Geometry: final body of the model. Coordinates: model frame, mm. A direction names the side the tool comes from. Give positions to 0.01 mm unless a question says otherwise; leave off trailing zeros. Loops run counter-clockwise (first coordinate to the right, second up) from the corner with the lowest first, then second, coordinate; pieces in that order, holes last. Notation, with made-up numbers: (-34, 59) -> (14, 59) arc R11 ccw to (14, 69) -> close; hole circle Ø7 at (-38, -27). An arc over 180 degrees is marked (long way). Answer in a Markdown table with one row per item. Add a question column.
from build123d import *

# Parameters (mm, degrees)
CYLINDER873_R               = 3.1
CYLINDER873_DEPTH           = 5
CYLINDER873_ROLL_ANGLE      = 90
CYLINDER872_R               = 5.6
CYLINDER872_DEPTH           = 4.5
CYLINDER872_ROLL_ANGLE      = 90
CYLINDER871_R               = 5.6
CYLINDER871_DEPTH           = 4
CYLINDER871_ROLL_ANGLE      = 90
CYLINDER870_R               = 3.5
CYLINDER870_DEPTH           = 14
CYLINDER870_ROLL_ANGLE      = 90
CYLINDER866_R               = 1.6
CYLINDER866_DEPTH           = 20
CYLINDER866_ROLL_ANGLE      = 90
CYLINDER869_R               = 2.1
CYLINDER869_DEPTH           = 20
CYLINDER869_ROLL_ANGLE      = 90
CYLINDER868_R               = 1.6
CYLINDER868_DEPTH           = 6.75
CYLINDER868_ROLL_ANGLE      = 90
CYLINDER867_R               = 2.8
CYLINDER867_DEPTH           = 10
CYLINDER867_ROLL_ANGLE      = 90
BOX542_W                    = 16
BOX542_H                    = 13
BOX542_DEPTH                = 14
BOX539_W                    = 12
BOX539_H                    = 7.5
BOX539_DEPTH                = 8
BOX538_W                    = 12
BOX538_H                    = 13.75
BOX538_DEPTH                = 12
BOX540_W                    = 30
BOX540_H                    = 3.75
BOX540_DEPTH                = 10
BOX541_W                    = 22
BOX541_H                    = 3.75
BOX541_DEPTH                = 14
FILLET352_R                 = 4
FILLET353_R                 = 3
FILLET354_R                 = 3
FILLET355_R                 = 4
FILLET356_R                 = 3
BOX543_W                    = 16
BOX543_H                    = 3.75
BOX543_DEPTH                = 2
CHAMFER102_SIZE             = 1.99
CYLINDER877_R               = 2.8
CYLINDER877_DEPTH           = 11
CYLINDER877_ROLL_ANGLE      = 89.99995
CYLINDER877_PITCH_ANGLE     = -5e-06
CYLINDER877_PLACEMENT_ANGLE = -10.999997
BOX545_W                    = 1.9
BOX545_H                    = 10
BOX545_DEPTH                = 8


with BuildPart() as cylinder1034:
    # Cylinder873 → Cylinder873 (new body)
    with BuildSketch(Plane.XY):
        Circle(CYLINDER873_R)
    extrude(amount=CYLINDER873_DEPTH)


with BuildPart() as cylinder1034_1:
    # Cylinder873 roll: moved
    add(cylinder1034.part.rotate(Axis((0, 0, 0), (1, 0, 0)), CYLINDER873_ROLL_ANGLE))


with BuildPart() as cylinder1034_2:
    # Cylinder873 placement: moved
    add(cylinder1034_1.part.moved(Location((49.5, 49.75, -13))))


with BuildPart() as cylinder1033:
    # Cylinder872 → Cylinder872 (new body)
    with BuildSketch(Plane.XY):
        Circle(CYLINDER872_R)
    extrude(amount=CYLINDER872_DEPTH)


with BuildPart() as cylinder1033_1:
    # Cylinder872 roll: moved
    add(cylinder1033.part.rotate(Axis((0, 0, 0), (1, 0, 0)), CYLINDER872_ROLL_ANGLE))


with BuildPart() as cylinder1033_2:
    # Cylinder872 placement: moved
    add(cylinder1033_1.part.moved(Location((38, 53.5, -11))))


with BuildPart() as cylinder1032:
    # Cylinder871 → Cylinder871 (new body)
    with BuildSketch(Plane.XY):
        Circle(CYLINDER871_R)
    extrude(amount=CYLINDER871_DEPTH)


with BuildPart() as cylinder1032_1:
    # Cylinder871 roll: moved
    add(cylinder1032.part.rotate(Axis((0, 0, 0), (1, 0, 0)), CYLINDER871_ROLL_ANGLE))


with BuildPart() as cylinder1032_2:
    # Cylinder871 placement: moved
    add(cylinder1032_1.part.moved(Location((38, 43.75, -11))))


with BuildPart() as fusion560:
    # Cylinder870 → Cylinder870 (new body)
    with BuildSketch(Plane.XY):
        Circle(CYLINDER870_R)
    extrude(amount=CYLINDER870_DEPTH)


with BuildPart() as fusion560_1:
    # Cylinder870 roll: moved
    add(fusion560.part.rotate(Axis((0, 0, 0), (1, 0, 0)), CYLINDER870_ROLL_ANGLE))


with BuildPart() as fusion560_2:
    # Cylinder870 placement: moved
    add(fusion560_1.part.moved(Location((38, 53.5, -11))))

    # Fusion560: union Cylinder1033, Cylinder1032
    add(cylinder1033_2.part)
    add(cylinder1032_2.part)


with BuildPart() as fusion560_3:
    # Fusion560 placement: moved
    add(fusion560_2.part.moved(Location((-1, 0, 0))))


with BuildPart() as cylinder1027:
    # Cylinder866 → Cylinder866 (new body)
    with BuildSketch(Plane.XY):
        Circle(CYLINDER866_R)
    extrude(amount=CYLINDER866_DEPTH)


with BuildPart() as cylinder1027_1:
    # Cylinder866 roll: moved
    add(cylinder1027.part.rotate(Axis((0, 0, 0), (1, 0, 0)), CYLINDER866_ROLL_ANGLE))


with BuildPart() as cylinder1027_2:
    # Cylinder866 placement: moved
    add(cylinder1027_1.part.moved(Location((49.5, 56.5, -13))))


with BuildPart() as cylinder1030:
    # Cylinder869 → Cylinder869 (new body)
    with BuildSketch(Plane.XY):
        Circle(CYLINDER869_R)
    extrude(amount=CYLINDER869_DEPTH)


with BuildPart() as cylinder1030_1:
    # Cylinder869 roll: moved
    add(cylinder1030.part.rotate(Axis((0, 0, 0), (1, 0, 0)), CYLINDER869_ROLL_ANGLE))


with BuildPart() as cylinder1030_2:
    # Cylinder869 placement: moved
    add(cylinder1030_1.part.moved(Location((45.5, 56.5, -26))))


with BuildPart() as fusion559:
    # Cylinder868 → Cylinder868 (new body)
    with BuildSketch(Plane.XY):
        Circle(CYLINDER868_R)
    extrude(amount=CYLINDER868_DEPTH)


with BuildPart() as fusion559_1:
    # Cylinder868 roll: moved
    add(fusion559.part.rotate(Axis((0, 0, 0), (1, 0, 0)), CYLINDER868_ROLL_ANGLE))


with BuildPart() as fusion559_2:
    # Cylinder868 placement: moved
    add(fusion559_1.part.moved(Location((28.5, 56.5, -11))))

    # Fusion559: union Cylinder1027, Cylinder1030
    add(cylinder1027_2.part)
    add(cylinder1030_2.part)


with BuildPart() as cylinder1028:
    # Cylinder867 → Cylinder867 (new body)
    with BuildSketch(Plane.XY):
        Circle(CYLINDER867_R)
    extrude(amount=CYLINDER867_DEPTH)


with BuildPart() as cylinder1028_1:
    # Cylinder867 roll: moved
    add(cylinder1028.part.rotate(Axis((0, 0, 0), (1, 0, 0)), CYLINDER867_ROLL_ANGLE))


with BuildPart() as cylinder1028_2:
    # Cylinder867 placement: moved
    add(cylinder1028_1.part.moved(Location((28.5, 49.75, -11))))


with BuildPart() as cube733:
    # Box542 → Box542 (new body)
    with BuildSketch(Plane(origin=(29.5, 39.75, -18), x_dir=(1, 0, 0), z_dir=(0, 0, 1))):
        with Locations((8, 6.5)):
            Rectangle(BOX542_W, BOX542_H)
    extrude(amount=BOX542_DEPTH)


with BuildPart() as cube730:
    # Box539 → Box539 (new body)
    with BuildSketch(Plane(origin=(389.5, 41.75, -32), x_dir=(1, 0, 0), z_dir=(0, 0, 1))):
        with Locations((6, 3.75)):
            Rectangle(BOX539_W, BOX539_H)
    extrude(amount=BOX539_DEPTH)


with BuildPart() as cut892:
    # Box538 → Box538 (new body)
    with BuildSketch(Plane(origin=(389.5, 39.75, -32), x_dir=(1, 0, 0), z_dir=(0, 0, 1))):
        with Locations((6, 6.875)):
            Rectangle(BOX538_W, BOX538_H)
    extrude(amount=BOX538_DEPTH)

    # Cut663: cut Cube730
    add(cube730.part, mode=Mode.SUBTRACT)


with BuildPart() as fusion556:
    # Box540 → Box540 (new body)
    with BuildSketch(Plane(origin=(373.5, 49.75, -20), x_dir=(1, 0, 0), z_dir=(0, 0, 1))):
        with Locations((15, 1.875)):
            Rectangle(BOX540_W, BOX540_H)
    extrude(amount=BOX540_DEPTH)

    # Fusion556: union Cut892
    add(cut892.part)


with BuildPart() as fusion556_1:
    # Fusion556 placement: moved
    add(fusion556.part.moved(Location((-350, 0, 2))))


with BuildPart() as fillet356:
    # Box541 → Box541 (new body)
    with BuildSketch(Plane(origin=(23.5, 49.75, -18), x_dir=(1, 0, 0), z_dir=(0, 0, 1))):
        with Locations((11, 1.875)):
            Rectangle(BOX541_W, BOX541_H)
    extrude(amount=BOX541_DEPTH)

    # Fusion557: union Fusion556
    add(fusion556_1.part)

    # Fusion558: union Cube733
    add(cube733.part)

    # Cut664: cut Cylinder1028
    add(cylinder1028_2.part, mode=Mode.SUBTRACT)

    # Cut665: cut Fusion559
    add(fusion559_2.part, mode=Mode.SUBTRACT)

    # Cut666: cut Fusion560
    add(fusion560_3.part, mode=Mode.SUBTRACT)

    # Fillet352
    fillet352_edges = [fillet356.edges().sort_by_distance(p)[0] for p in [
        (51.5, 40.75, -30),
        (51.5, 51.375, -30),
        (39.5, 40.75, -30),
        (39.5, 51.375, -30),
    ]]
    fillet(fillet352_edges, radius=FILLET352_R)

    # Fillet353
    fillet353_edges = [fillet356.edges().sort_by_distance(p)[0] for p in [
        (49.5, 49.75, -8),
        (48.5, 39.75, -18),
    ]]
    fillet(fillet353_edges, radius=FILLET353_R)

    # Fillet354
    fillet354_edges = [fillet356.edges().sort_by_distance(p)[0] for p in [
        (48.5, 49.75, -18),
    ]]
    fillet(fillet354_edges, radius=FILLET354_R)

    # Cut667: cut Cylinder1034
    add(cylinder1034_2.part, mode=Mode.SUBTRACT)

    # Fillet355
    fillet355_edges = [fillet356.edges().sort_by_distance(p)[0] for p in [
        (23.5, 51.625, -18),
        (23.5, 51.625, -4),
    ]]
    fillet(fillet355_edges, radius=FILLET355_R)

    # Fillet356
    fillet356_edges = [fillet356.edges().sort_by_distance(p)[0] for p in [
        (29.5, 44.75, -18),
        (45.5, 46.625, -4),
        (29.5, 44.75, -4),
    ]]
    fillet(fillet356_edges, radius=FILLET356_R)


with BuildPart() as chamfer102:
    # Box543 → Box543 (new body)
    with BuildSketch(Plane(origin=(37.5, 49.75, -20), x_dir=(1, 0, 0), z_dir=(0, 0, 1))):
        with Locations((8, 1.875)):
            Rectangle(BOX543_W, BOX543_H)
    extrude(amount=BOX543_DEPTH)

    # Chamfer102
    chamfer102_edges = [chamfer102.edges().sort_by_distance(p)[0] for p in [
        (37.5, 51.625, -20),
        (53.5, 51.625, -20),
    ]]
    chamfer(chamfer102_edges, length=CHAMFER102_SIZE)


with BuildPart() as cylinder1038:
    # Cylinder877 → Cylinder877 (new body)
    with BuildSketch(Plane.XY):
        Circle(CYLINDER877_R)
    extrude(amount=CYLINDER877_DEPTH)


with BuildPart() as cylinder1038_1:
    # Cylinder877 roll: moved
    add(cylinder1038.part.rotate(Axis((0, 0, 0), (1, 0, 0)), CYLINDER877_ROLL_ANGLE))


with BuildPart() as cylinder1038_2:
    # Cylinder877 pitch: moved
    add(cylinder1038_1.part.rotate(Axis((0, 0, 0), (0, 1, 0)), CYLINDER877_PITCH_ANGLE))


with BuildPart() as cylinder1038_3:
    # Cylinder877 placement: moved
    add(cylinder1038_2.part.moved(Location((29.8503, 50.5822, -11))).rotate(Axis((29.8503, 50.5822, -11), (0, 0, 1)), CYLINDER877_PLACEMENT_ANGLE))


with BuildPart() as obj1:
    # Box545 → Box545 (new body)
    with BuildSketch(Plane(origin=(29.5, 39.75, -15), x_dir=(1, 0, 0), z_dir=(0, 0, 1))):
        with Locations((0.95, 5)):
            Rectangle(BOX545_W, BOX545_H)
    extrude(amount=BOX545_DEPTH)

    # Cut669: cut Cylinder1038
    add(cylinder1038_3.part, mode=Mode.SUBTRACT)

    # Fusion563: union Fillet356, Chamfer102
    add(fillet356.part)
    add(chamfer102.part)


solid = obj1.part
(1) Draft query along Z for faces 1 (the flat face through (35, 48, -18)), 2 (the flat face through (29.5, 45, -8)), 3 (the cylindrical face through (31.405, 41.778, -10.754)). Return one class per face: +Z half, -Z half, draft (parallel to the pull), parting line (faces both ways), or undercut.
(2) Cut plane C-C on x = 28.5. Return the cut outline in (y, z).
(3) Reachability of faces 4 (the cylindrical face through (30.4, 44.82, -4.86)), 5 (the flat face through (44, 49.25, -24)), 6 (the cylindrical face through (48.54, 40.61, -18.9)), 7 (the flat face through (37, 43.75, -15)) from +Z, -Z, +X, -X, +Y, -Y: full face, straight path, thin tool, end or side. Return the list, or none.
(4) Cut plane D-D on z = -19.5. Return the cut outline in (x, y).
(5) Material intervals for line 1 along Z through (x, y) = (37, 51.4); line 2 along Y through (x, z) = (39.75, -24.25); line 3 along X through (y, z) = (40.65, -26), sorted ascending. Write a range as from..to.
(6) Cut plane A-A on x = 37. Return the cut outline in (y, z), then the cut area to 4 significant figures.
(7) Pin query (flat end, axial travel): pin 1 Ø2 at (y, z) = (48, -8) entering from +X; pin 2 Ø1 at (y, z) = (42, -26) entering from +X; pin 3 Ø5 at (x, y) = (34, 47) entering from -Z; pin 4 Ø6.5 at (x, z) = (45.5, -27) entering from -Y. Return the tip coordinate at first contact, or that it passes through.
(8) Cut plane B-B on y = 45.75. Return the cut outline in (x, z), then the cut area to 3 significant figures.
Answer list:
| question | item | result |
|---|---|---|
| 1 | face 1 | -Z half |
| 1 | face 2 | draft |
| 1 | face 3 | undercut |
| 2 | outline | (49.75, -18) -> (53.5, -18) -> (53.5, -12.6) -> (49.75, -12.6) -> close; (49.75, -9.4) -> (53.5, -9.4) -> (53.5, -4) -> (49.75, -4) -> close |
| 3 | face 4 | +Z, -X, -Y |
| 3 | face 5 | -Z, +X, -X |
| 3 | face 6 | +Z, +X, -Y |
| 3 | face 7 | -Y |
| 4 | outline | (38.99, 49.75) -> (39.5, 49.75) -> (39.5, 39.75) -> (45.5, 39.75) -> (45.5, 40.15) -> (51.5, 40.15) -> (51.5, 49.75) -> (52.01, 49.75) -> (52.01, 53.5) -> (38.99, 53.5) -> close |
| 5 | line 1 | z = -18..-16.6, -5.4..-4 |
| 5 | line 2 | y = 39.75..41.75, 49.25..53.5 |
| 5 | line 3 | x = 39.5..43.4, 47.6..51.5 |
| 6 | outline | (39.75, -18) -> (53.5, -18) -> (53.5, -16.6) -> (49, -16.6) -> (49, -14.5) -> (43.75, -14.5) -> (43.75, -16.6) -> (39.75, -16.6) -> close; (39.75, -5.4) -> (43.75, -5.4) -> (43.75, -7.5) -> (49, -7.5) -> (49, -5.4) -> (53.5, -5.4) -> (53.5, -4) -> (39.75, -4) -> close |
| 6 | area | 60.55 mm² |
| 7 | pin 1 | stops at x = 45.5 |
| 7 | pin 2 | stops at x = 51.5 |
| 7 | pin 3 | stops at z = -18 |
| 7 | pin 4 | stops at y = 39.75 |
| 8 | outline | (29.5, -15) arc R3 ccw to (32.5, -18) -> (39.5, -18) -> (39.5, -22) -> (51.5, -22) -> (51.5, -18) -> (45.5, -18) -> (45.5, -7) arc R3 ccw to (42.5, -4) -> (32.5, -4) arc R3 ccw to (29.5, -7) -> (29.5, -8.38) arc R2.8 cw to (29.5, -13.62) -> close; hole circle Ø7 at (37, -11) |
| 8 | area | 221 mm² |
